Could you check a few things on this model? Use its own coordinates, in mm. Face numbers are marked on the shaded views. A direction names the side the tool comes from. Give positions to 0.01 mm unless a question says otherwise; leave off trailing zeros. Loops run counter-clockwise (first coordinate to the right, second up) from the corner with the lowest first, then second, coordinate; pieces in that order, holes last. Notation, with made-up numbers: (14, 71.5) - (20, 71.5) arc R12 cw to (20, 84.5) - close; hole circle Ø8 at (-9, -5). An arc over 180 degrees is marked (long way). Use CSV: the item, a comma, the result in double quotes.
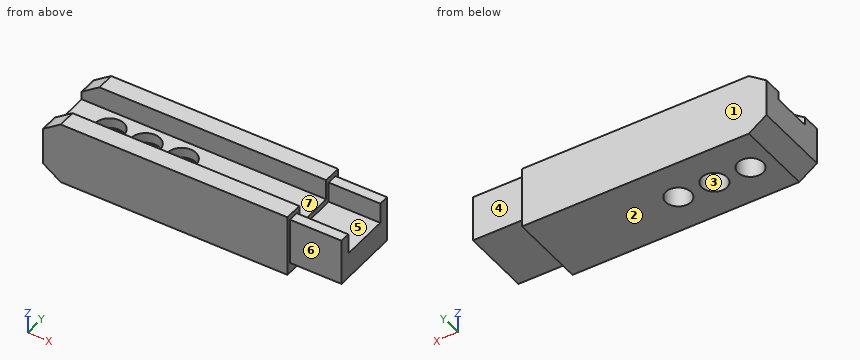
Autodesk Inventor part; units mm, degrees
ref_plane "YZ Plane" through (0, 0, 0) normal (1, 0, 0) x (0, 1, 0)
ref_plane "XZ Plane" through (0, 0, 0) normal (0, 1, 0) x (-1, 0, 0)
ref_plane "XY Plane" through (0, 0, 0) normal (0, 0, 1) x (1, 0, 0)
sketch "Náčrt1" plane through (0, 0, 0) normal (0, 1, 0) x (-1, 0, 0)
  line L0 (0, 0) -> (50, 0)
  line L1 (50, 0) -> (66.0697, -19.1511)
  line L2 (50, 0) -> (75, 0) construction
  line L3 (66.0697, -19.1511) -> (58.4092, -25.579)
  line L4 (0, -12) -> (0, 0)
  line L5 (58.6554, -25.3724) -> (47.4347, -12)
  line L6 (47.4347, -12) -> (0, -12)
  dimension "d0" = 50
  dimension "d2" = 25
  dimension "d3" = 50
  dimension "d4" = 10
  dimension "d5" = 12
extrude "Vysunutí1" add sketch "Náčrt1" along normal blind 15
sketch "Náčrt11" plane through (0, 0, 0) normal (1, 0, 0) x (0, 0, -1)
  line L0 (0, 0) -> (0, 15)
  line L1 (0, 7.5) -> (12, 7.5)
  line L2 (12, 0) -> (12, 15)
  line L3 (0, 3.5) -> (4, 3.5)
  line L4 (4, 3.5) -> (4, 11.5)
  line L5 (4, 11.5) -> (0, 11.5)
  line L6 (0, 11.5) -> (0, 3.5)
  point P0 (0, 7.5)
  point P1 (0, 11.5)
  dimension "d64" = 4
  dimension "d65" = 8
extrude "Vysunutí10" cut sketch "Náčrt11" against normal through all
sketch "Náčrt21" plane through (-66.0697, 0, -19.1511) normal (-0.6428, 0, -0.766) x (-0.766, 0, 0.6428)
  line L0 (0, 0) -> (0, 15)
  line L1 (0, 3.5) -> (-4, 3.5)
  line L2 (-4, 3.5) -> (-4, 11.5)
  line L3 (-4, 11.5) -> (0, 11.5)
  line L4 (0, 11.5) -> (0, 3.5)
  point P0 (-38.3022, 0)
  point P1 (0, 7.5)
  point P2 (0, 11.5)
  dimension "d68" = 4
  dimension "d69" = 8
extrude "Vysunutí11" cut sketch "Náčrt21" against normal through all
sketch "Náčrt30" plane through (0, 0, -12) normal (0, 0, -1) x (-1, 0, 0)
  point P0 (0, 0)
sketch "Náčrt31" plane through (0, 0, 0) normal (1, 0, 0) x (0, 0, -1)
  point P0 (0, 0)
sketch "Náčrt32" plane through (0, 0, 0) normal (0, -1, 0) x (1, 0, 0)
  line L0 (-47.4347, -12) -> (-58.6554, -25.3724)
  line L1 (-47.4347, -12) -> (-47.4347, 0)
  line L2 (-47.4347, -12) -> (-58.6554, -25.3724)
  line L3 (-58.6554, -25.3724) -> (-66.0697, -19.1511)
  line L4 (-66.0697, -19.1511) -> (-50, 0)
  line L5 (-50, 0) -> (-47.4347, 0)
  line L6 (-50, 0) -> (0, 0)
  point P0 (-47.4347, 0)
extrude "Vysunutí16" add sketch "Náčrt32" against normal through all
sketch "Náčrt33" plane through (0, 0, 0) normal (0, -1, 0) x (1, 0, 0)
  line L0 (-47.4347, -12) -> (-58.6554, -25.3724)
  line L1 (-47.4347, -4) -> (-47.4347, 0)
  line L2 (-47.4347, -12) -> (-47.4347, 0)
  line L3 (-66.0697, -19.1511) -> (-50, 0)
  line L4 (-47.4347, 0) -> (-50, 0)
  line L5 (-50, 0) -> (-66.0697, -19.1511)
  line L6 (-50, 0) -> (0, 0)
  line L7 (-66.0697, -19.1511) -> (-50, 0)
  line L8 (-58.6554, -25.3724) -> (-66.0697, -19.1511)
  line L9 (-47.4347, -12) -> (-58.6554, -25.3724)
  line L10 (0, -12) -> (-47.4347, -12)
  line L11 (0, 0) -> (0, -12)
  line L12 (-58.6554, -25.3724) -> (-66.0697, -19.1511)
  line L13 (-66.0697, -19.1511) -> (-58.6554, -25.3724)
  line L14 (-58.6554, -25.3724) -> (-47.4347, -12)
extrude "Vysunutí17" cut sketch "Náčrt33" against normal through all contours L0 L8 L3 L4 L1 L2
sketch "Náčrt34" plane through (0, 0, 0) normal (0, -1, 0) x (1, 0, 0)
  line L0 (-47.4347, 0) -> (-47.4347, -12)
  line L1 (-47.4347, 0) -> (-47.4347, -12)
  line L2 (0, -12) -> (-47.4347, -12)
  line L3 (0, 0) -> (0, -12)
  line L4 (-47.4347, 0) -> (0, 0)
  line L5 (0, -12) -> (-47.4347, -12)
  line L6 (-44, -12) -> (-47.4347, -9.595)
  line L7 (-44, -12) -> (-39.807, -12) construction
  line L8 (-47.4347, -9.595) -> (-47.4347, -12)
  line L9 (-44, -12) -> (-47.4347, -12)
  line L10 (0, 0) -> (-47.4347, 0)
  line L11 (-44, 0) -> (-47.0563, -2.14)
  line L12 (-44, 0) -> (-40.269, 0) construction
  line L13 (-47.0563, -2.14) -> (-47.4347, -2.405)
  line L14 (-47.4347, -2.405) -> (-47.4347, 0)
  line L15 (-44, 0) -> (-47.4347, 0)
  dimension "d99" = 145
  dimension "d100" = 145
extrude "Vysunutí18" cut sketch "Náčrt34" against normal through all contours L4 L11 L13 L0 | L6 L2 L0
sketch "Náčrt35" plane through (0, 3.5, -4) normal (0, 0, 1) x (1, 0, 0)
  line L0 (-47.4347, 8) -> (-47.4347, 0)
  line L1 (-47.4347, 4) -> (0, 4)
  line L2 (0, 10.8249) -> (0, -2.8249)
  circle A0 centre (-39.435, 4) radius 2.8
  circle A1 centre (-32.435, 4) radius 2.8
  circle A2 centre (-25.435, 4) radius 2.8
  point P0 (0, -3.5)
  dimension "d103" = 5.6
  dimension "d104" = 5.6
  dimension "d105" = 5.6
extrude "Vysunutí19" cut sketch "Náčrt35" against normal blind 2
sketch "Náčrt36" plane through (-39.435, 7.5, -6) normal (0, 0, 1) x (1, 0, 0)
  circle A0 centre (0, 0) radius 2.45
  point P0 (39.435, -7.5)
  dimension "d108" = 4.9
sketch "Náčrt37" plane through (-32.435, 7.5, -6) normal (0, 0, 1) x (1, 0, 0)
  circle A0 centre (0, 0) radius 2.45
  point P0 (32.435, -7.5)
  dimension "d109" = 4.9
sketch "Náčrt38" plane through (-25.435, 7.5, -6) normal (0, 0, 1) x (1, 0, 0)
  circle A0 centre (0, 0) radius 2.45
  point P0 (25.435, -7.5)
  dimension "d110" = 4.9
extrude "Vysunutí20" cut sketch "Náčrt36" against normal through all
extrude "Vysunutí21" cut sketch "Náčrt37" against normal through all
sketch "Náčrt39" plane through (0, 0, 0) normal (1, 0, 0) x (0, 0, -1)
  line L0 (0, 11.5) -> (0, 15)
  line L1 (12, 0) -> (12, 15)
  line L2 (0, 0) -> (0, 3.5)
  line L3 (1, 0.75) -> (10, 0.75)
  line L4 (10, 14.25) -> (1, 14.25)
  line L5 (1, 14.25) -> (1, 12.2503)
  line L6 (4, 4.7) -> (4, 10.3)
  line L7 (5, 12.2503) -> (1, 12.2503)
  line L8 (1, 0.75) -> (1, 2.7496)
  line L9 (1, 2.7496) -> (5, 2.7496)
  line L10 (5, 2.7496) -> (5, 12.2503)
  line L11 (10, 0.75) -> (10, 14.25)
  line L12 (4, 7.5) -> (12, 7.5)
  line L13 (12, 9.95) -> (12, 5.05)
  point P0 (1, 1.7498)
  point P1 (5, 7.5)
  point P2 (1, 13.2502)
  point P3 (10, 7.5)
  point P4 (5.5, 0.75)
  dimension "d119" = 13.5
extrude "Vysunutí22" add sketch "Náčrt39" along normal blind 10
extrude "Vysunutí23" cut sketch "Náčrt38" against normal through all
properties part number "SEMAFOR1"
1) I need wall thicknesses on line 1 along X through (y, z) = (7.5, -4.5) (3 decimals); line 2 along X through (y, z) = (7.5, -5.6) (3 decimals); line 3 along Y through (x, z) = (-39.5, -2.75). Which ranges of each line are inside material? Lowest first, please.
Answer below:
line 1,"x = -47.435 to -42.235, -36.635 to -35.235, -29.635 to -28.235, -22.635 to 0"
line 2,"x = -47.435 to -42.235, -36.635 to -35.235, -29.635 to -28.235, -22.635 to 10"
line 3,"y = 0 to 3.5, 11.5 to 15"
2) I'm going to push flat-ended pins straight in: P1, Ø3, axis at x = -40, y = 7.5, coming from the +Z side; P2, Ø3, axis at x = -12, z = -3, coming from the -Y side; P3, Ø2.5, axis at x = 6, z = -3.5, coming from the +Y side; P4, Ø0.6, axis at x = 6.5, y = 13.5, coming from the +Z side. Where does each tip first touch, or does it pass through?
Answer below:
P1,"passes through"
P2,"stops at y = 0"
P3,"stops at y = 14.25"
P4,"stops at z = -1"
3) We'd pull the mould along Y, two halves only. Please class the marked faces 1, 2 and 3: +Y half, -Y half, draft (parallel to the pull), parting line (faces both ways), or undercut.
Answer below:
face 1,"+Y half"
face 2,"draft"
face 3,"undercut"
4) Suppose I cut it at A-A (y = 7.5). State how many separate pieces and enclosed holes the cut face has, plus the area to 3 significant figures.
Answer below:
separate pieces,"4"
enclosed holes,"0"
area,"304 mm2"
5) Suppose I cut it at C-C (x = -39). Please give me the cut outline in (y, z), plus the area to 3 significant figures.
Answer below:
outline,"(0, -12) - (5.09, -12) - (5.09, -6) - (4.73, -6) - (4.73, -4) - (3.5, -4) - (3.5, 0) - (0, 0) - close; (9.91, -12) - (15, -12) - (15, 0) - (11.5, 0) - (11.5, -4) - (10.27, -4) - (10.27, -6) - (9.91, -6) - close"
area,"108 mm2"
6) Which directions (+Z, -Z, +X, -X, +Y, -Y) give clear straight access to the entire face, cutting with the end or side of a thin tool? Please do the marked faces 4, 5, 6 and 7.
Answer below:
face 4,"+Z, -Z, +X, +Y"
face 5,"+Z, +X"
face 6,"+Z, -Z, +X, -Y"
face 7,"+Z, +X, -X"
7) Suppose I cut it at D-D (z = -1.5). Please give me the cut outline in (x, y), plus the area to 3 significant figures.
Answer below:
outline,"(-46.14, 0) - (0, 0) - (0, 0.75) - (10, 0.75) - (10, 2.75) - (0, 2.75) - (0, 3.5) - (-46.14, 3.5) - close; (-46.14, 11.5) - (0, 11.5) - (0, 12.25) - (10, 12.25) - (10, 14.25) - (0, 14.25) - (0, 15) - (-46.14, 15) - close"
area,"363 mm2"
8) Suppose I cut it at B-B (z = -7.25). Please give me the cut outline in (x, y) (3 decimals).
Answer below:
outline,"(-47.435, 0) - (0, 0) - (0, 0.75) - (10, 0.75) - (10, 14.25) - (0, 14.25) - (0, 15) - (-47.435, 15) - close; hole circle Ø4.9 at (-39.435, 7.5); hole circle Ø4.9 at (-32.435, 7.5); hole circle Ø4.9 at (-25.435, 7.5)"
